from build123d import *

# Parameters (mm, degrees)
F1_DEPTH      = 3.175
F1_DEPTH_BACK = 3.175
F2_DEPTH      = 6.35
F2_DEPTH_BACK = 6.35
F3_SIZE       = 6.34999
F4_R          = 5.715
F5_R          = 0.635


# Not quite as in the source:
# - a fillet or chamfer is up to 0.001 mm smaller than in the source, because OpenCascade refuses the exact size


with BuildPart() as f1:
    # F0 (on Top) → F1 (new body, two sides)
    with BuildSketch(Plane.XY) as f1_sk:
        Polygon((-41.6700830699, 59.9633481442), (-41.6700830699, -6.6100518558), (-32.9213373307, -6.9480776483), (-32.9213373307, 51.4719223517), align=None)
    extrude(amount=F1_DEPTH)
    extrude(f1_sk.sketch, amount=-F1_DEPTH_BACK)

    # F0 (on Top) → F2 (join, two sides)
    with BuildSketch(Plane.XY) as f2_sk:
        Polygon((-32.9213373307, -6.9480776483), (-41.6700830699, -6.6100518558), (-46.7643177352, -6.4132256179), (-46.7643177352, -10.747612454), (-41.6700830699, -10.9444386919), (-41.6700830699, -40.1244200766), (-31.2753289716, -40.5260427889), (-31.2753289716, -11.7029547691), (-25.3439064165, -11.9321274837), (-25.3439064165, -6.6100518558), align=None)
    extrude(amount=F2_DEPTH)
    extrude(f2_sk.sketch, amount=-F2_DEPTH_BACK)

    # F3 (size 6.35 in the source; OpenCascade refuses exactly that, so slightly less here)
    f3_edges = [f1.edges().sort_by_distance(p)[0] for p in [
        (-32.921337, 22.261922, 3.175),
    ]]
    chamfer(f3_edges, length=F3_SIZE)

    # F4 (call 1 of 4: OpenCascade refuses the feature's edges together)
    f4_edges = [f1.edges().sort_by_distance(p)[0] for p in [
        (-31.275329, -26.114499, 6.35),
    ]]
    fillet(f4_edges, radius=F4_R)

    # F4#2 (call 2 of 4)
    f4_2_edges = [f1.edges().sort_by_distance(p)[0] for p in [
        (-41.670083, -25.534429, 6.35),
    ]]
    fillet(f4_2_edges, radius=F4_R)

    # F4#3 (call 3 of 4)
    f4_3_edges = [f1.edges().sort_by_distance(p)[0] for p in [
        (-31.275329, -26.114499, -6.35),
    ]]
    fillet(f4_3_edges, radius=F4_R)

    # F4#4 (call 4 of 4)
    f4_4_edges = [f1.edges().sort_by_distance(p)[0] for p in [
        (-41.670083, -25.534429, -6.35),
    ]]
    fillet(f4_4_edges, radius=F4_R)

    # F5
    f5_edges = [f1.edges().sort_by_distance(p)[0] for p in [
        (-41.670083, 26.676648, 3.175),
    ]]
    fillet(f5_edges, radius=F5_R)


solid = f1.part
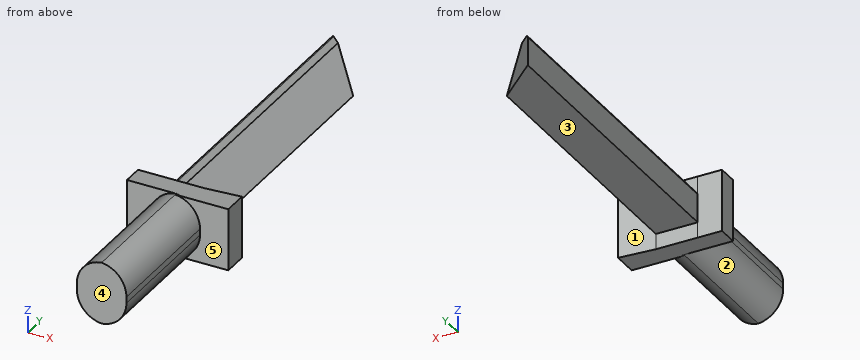
Read the model definition and answer for the solid it produces. Units are mm, in the model's axes. Face numbers are marked on the shaded views. A direction names the side the tool comes from. Round coordinates to 2 decimals unless told otherwise and drop trailing zeros. Loops run counter-clockwise (first coordinate to the right, second up) from the corner with the lowest first, then second, coordinate; pieces in that order, holes last. Notation, with made-up numbers: (-2, 86.5) - (28, 86.5) arc R11 ccw to (28, 93.5) - close; hole circle Ø4 at (-16.5, 69). An arc over 180 degrees is marked (long way). One line per question, with ' | ' between items. Start each with the question number.
Q1. Section D-D on y = -15 is taken. Give the vertices of the cut face in (x, z) (3 decimals).
Q2. For a pull along X with two mould halves and no side action, classify the marked faces 3, 4 and 5 as +X half, -X half, draft (parallel to the pull), parting line (faces both ways), or undercut.
Q3. Find the intervals of material crossed by L1, parallel to Z at x = -40, y = 10.5 (3 decimals); L2, parallel to X at y = -33, z = -5; L3, parallel to Z at x = -32.25, y = -28, in increasing order.
Q4. Section A-A on z = -4.75 is taken. Give the vertices of the cut face in (x, y), plus the area to 3 significant figures.
Q5. Flat-ended cylindrical pins translate along their axes: pin 1 (1 mm diameter, centred on x = -33.5, z = 2.5, fed in from -Y); pin 2 (5 mm diameter, centred on y = 9, z = 3, fed in from -X); pin 3 (2.5 mm diameter, centred on x = -36, y = 24.5, fed in from -Z) (3 decimals). Find the tip coordinate at first contact, or state that the pin passes through.
Q6. For the marked faces 1 and 2, determine the directions among +Z, -Z, +X, -X, +Y, -Y from which every point of the face is accessible in a straight line to the end or side of a thin tool.
Q7. Section C-C on x = -34.75 is taken. Give the vertices of the cut face in (y, z) (3 decimals).
Established:
1) outline: (-41.67, -0.635) arc R5.715 ccw to (-36.473, -6.327) arc R5.715 ccw to (-31.275, -0.635) - (-31.275, 0.635) arc R5.715 ccw to (-36.473, 6.327) arc R5.715 ccw to (-41.67, 0.635) - close
2) face 3: draft | face 4: -X half | face 5: undercut
3) L1: -3.175 to 3.175 | L2: -39.64 to -33.3 | L3: -3.83 to 3.83
4) outline: (-46.76, -10.75) - (-39.92, -11.01) - (-39.92, -40.19) - (-33.02, -40.46) - (-33.02, -11.64) - (-25.34, -11.93) - (-25.34, -6.61) - (-32.92, -6.95) - (-46.76, -6.41) - close | area: 299 mm²
5) pin 1: y = -40.46 | pin 2: x = -41.67 | pin 3: z = -3.175
6) face 1: +Z, -Z, +Y | face 2: -Z, -X, -Y
7) outline: (-40.392, -5.893) - (-11.569, -5.893) - (-11.569, -6.35) - (-6.877, -6.35) - (-6.877, -3.175) - (53.247, -3.175) - (53.247, -1.346) - (-6.877, -1.346) - (-6.877, 6.35) - (-11.569, 6.35) - (-11.569, 5.893) - (-40.392, 5.893) - close
